from build123d import *


with BuildPart() as f1:
    # F0 (on Front) → F1 (revolve)
    with BuildSketch(Plane.XZ):
        Polygon((-11.17308, 3.4), (-11.17308, 0), (17.72692, 0), (17.72692, 2.6), (-4.27308, 2.6), (-4.27308, 3.4), align=None)
        Polygon((17.72692, 2.6), (17.72692, 0), (18.72692, 0), (18.72692, 3.5), (17.72692, 3.5), align=None)
    revolve(axis=Axis((2.68319, 0, 0), (1, 0, 0)))

    # F2 (on Front) → F3 (revolve, cut)
    with BuildSketch(Plane.XZ):
        Polygon((-12.316774, 2.9), (-12.316774, 0), (20.493909, 0), (20.493909, 2), (-4.616774, 2), (-4.616774, 2.9), align=None)
    revolve(axis=Axis((3.41996, 0, 0), (1, 0, 0)), mode=Mode.SUBTRACT)


solid = f1.part
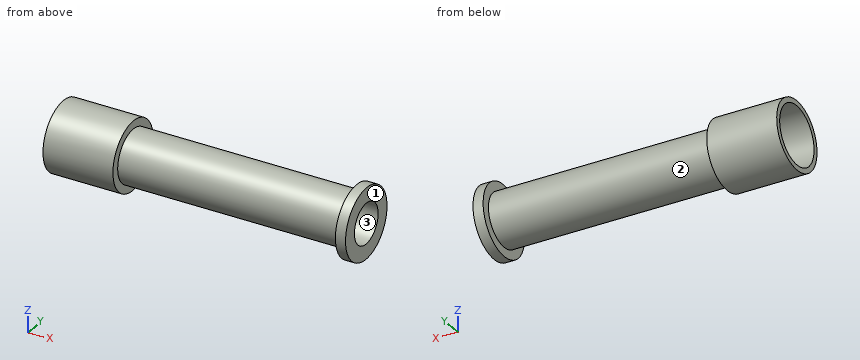
Build history of the part. All positions in model axes, mm. Face numbers are marked on the shaded views. Coordinates: 2 decimals unless noted, no trailing zeros. Write each loop counter-clockwise with the first axis right and the second up, starting at its lowest first coordinate (ties: lowest second). Pieces come first, ordered by that corner, then holes.
(1) Cut at A-A on z = 0. List the corners of the cut face in (x, y).
(2) Cut at B-B on y = -0.5. List the corners of the cut face in (x, z), and give its area (3 significant figures).
(3) Pin check, flat tips, straight feed: pin 1 Ø1.7 at (y, z) = (1, -0.5) entering from -X; pin 2 Ø1 at (x, z) = (11.5, -2) entering from +Y; pin 3 Ø1 at (x, z) = (8, -2.5) entering from -Y; pin 4 Ø2 at (x, z) = (13, -0.5) entering from -Y. Stop position of each tip, or through.
(4) Cut at C-C on x = 3.25. List the corners of the cut face in (y, z).
(5) Drill centre lines: line 1 (X direction, y = -1, z = 3); line 2 (Y direction, x = 11.75, z = 0); line 3 (Y direction, x = -7.75, z = 0). Where is each one in solid material? Low to high.
(6) Mould opens along Y. For the marked faces 1, 2 and 3 say: pulls with the +Y half, pulls with the -Y half, needs draft (parallel to the pull), parting line crosses it, or undercut.
Working result:
1. outline: (-11.17, -3.4) - (-4.27, -3.4) - (-4.27, -2.6) - (17.73, -2.6) - (17.73, -3.5) - (18.73, -3.5) - (18.73, -2) - (-4.62, -2) - (-4.62, -2.9) - (-11.17, -2.9) - close; (-11.17, 2.9) - (-4.62, 2.9) - (-4.62, 2) - (18.73, 2) - (18.73, 3.5) - (17.73, 3.5) - (17.73, 2.6) - (-4.27, 2.6) - (-4.27, 3.4) - (-11.17, 3.4) - close
2. outline: (-11.17, -3.36) - (-4.27, -3.36) - (-4.27, -2.55) - (17.73, -2.55) - (17.73, -3.46) - (18.73, -3.46) - (18.73, -1.94) - (-4.62, -1.94) - (-4.62, -2.86) - (-11.17, -2.86) - close; (-11.17, 2.86) - (-4.62, 2.86) - (-4.62, 1.94) - (18.73, 1.94) - (18.73, 3.46) - (17.73, 3.46) - (17.73, 2.55) - (-4.27, 2.55) - (-4.27, 3.36) - (-11.17, 3.36) - close
2. area: 37.7 mm2
3. pin 1: passes through
3. pin 2: stops at y = 2.12
3. pin 3: stops at y = -1.66
3. pin 4: stops at y = -2.6
4. outline: circle Ø5.2 at (0, 0); hole circle Ø4 at (0, 0)
5. line 1: x = -11.17 to -4.27, 17.73 to 18.73
5. line 2: y = -2.6 to -2, 2 to 2.6
5. line 3: y = -3.4 to -2.9, 2.9 to 3.4
6. face 1: needs draft
6. face 2: parting line crosses it
6. face 3: undercut
